Read the model definition and answer for the solid it produces. Units are mm, in the model's axes. A direction names the side the tool comes from. Round coordinates to 2 decimals unless told otherwise and drop trailing zeros. Order: outer loops, then holes, each group sorted by start corner. A loop starts at its lowest first (then second) coordinate and runs counter-clockwise, first axis right, second up. Notation, with made-up numbers: (-19, 12) - (35, 12) arc R25 ccw to (35, 37) - close; hole circle Ø8 at (8.5, 33). An arc over 180 degrees is marked (long way). Put each result on its own line as item: value. Start each with the question number.
Q1. Each of these flat-tipped pins is pushed along its axis until it touches: pin 1 Ø2.5 at (x, z) = (98, 2.5) entering from +Y (3 decimals); pin 2 Ø12 at (x, z) = (28.575, 44.45) entering from -Y; pin 3 Ø6.5 at (x, z) = (89.5, 5) entering from -Y (3 decimals); pin 4 Ø8 at (y, z) = (82, 16) entering from +X. Where does it stop, or does it pass through?
Q2. Section C-C on x = 81 is taken. Give the vertices of the cut face in (y, z) (1 decimal).
Q3. Which of the six approach directions +Z, -Z, +X, -X, +Y, -Y give full straight-line access (tool end or side, diameter ignored) to faces 1 (the face through (28.175, 79.514, 9.465)), 2 (the face through (88, 66.675, 4)), 3 (the face through (87, 22.225, 4))?
Q4. Section A-A on z = 29.5 is taken. Give the vertices of the cut face in (x, y), then the cut area to 3 significant figures.
Q5. For a pull along X with two mould halves and no side action, classify faces 4 (the face through (57.15, 6, 17)), 5 (the face through (29, 88.9, 29)), 6 (the face through (64.83, 38.17, 3.91)), 7 (the face through (27.95, 4.02, 73.02)) as pulls with the +X half, pulls with the -X half, needs draft (parallel to the pull), parting line crosses it, or undercut.
Q6. Find the intervals of material crossed by line 1 along X through (y, z) = (44, 3); line 2 along X through (y, z) = (3, 44); line 3 along Y through (x, z) = (18, 52.5), in increasing order. Write a range as from..to.
Q7. Section D-D on y = 44.45 is taken. Give the vertices of the cut face in (x, z), then the cut area to 3 significant figures.
from build123d import *

# Parameters (mm, degrees)
F0_W     = 57.15
F0_H     = 7.9375
F0_R     = 10.3251
F1_DEPTH = 7.9375
F2_DEPTH = 44.45
F3_DEPTH = 44.45
F4_W     = 28.575
F4_H     = 7.9375
F6_W     = 28.575
F6_H     = 7.9375
F8_R     = 9.92251
F9_DEPTH = 88.901
F10_R    = 5.08


with BuildPart() as f1:
    # F0 (on Top) → F1 (new body)
    with BuildSketch(Plane.XY):
        with Locations((28.575, 3.96875)):
            Rectangle(F0_W, F0_H)
        with BuildLine():
            Line((0, 80.9625), (0, 7.9375))
            Line((0, 7.9375), (57.15, 7.9375))
            Line((57.15, 7.9375), (57.15, 15.875))
            ThreePointArc((57.15, 15.875), (59.009872, 20.365128), (63.5, 22.225))
            Line((63.5, 22.225), (111.125, 22.225))
            ThreePointArc((111.125, 22.225), (133.35, 44.45), (111.125, 66.675))
            Line((111.125, 66.675), (63.5, 66.675))
            ThreePointArc((63.5, 66.675), (59.009872, 68.534872), (57.15, 73.025))
            Line((57.15, 73.025), (57.15, 80.9625))
            Line((57.15, 80.9625), (0, 80.9625))
        make_face()
        with Locations((73.025, 44.45)):
            Circle(F0_R, mode=Mode.SUBTRACT)
        with Locations((111.125, 44.45)):
            Circle(F0_R, mode=Mode.SUBTRACT)
        with Locations((28.575, 84.93125)):
            Rectangle(F0_W, F0_H)
    extrude(amount=F1_DEPTH)

    # F0 (on Top) → F2 (join)
    with BuildSketch(Plane.XY):
        with Locations((28.575, 3.96875)):
            Rectangle(F0_W, F0_H)
    extrude(amount=F2_DEPTH)

    # F0 (on Top) → F3 (join)
    with BuildSketch(Plane.XY):
        with Locations((28.575, 84.93125)):
            Rectangle(F0_W, F0_H)
    extrude(amount=F3_DEPTH)

    # F4 (on face) → F5 (revolve)
    with BuildSketch(Plane.XY.offset(44.45)):
        with Locations((14.2875, 3.96875)):
            Rectangle(F4_W, F4_H)
    revolve(axis=Axis((28.575, 3.96875, 44.45), (0, 1, 0)))

    # F6 (on face) → F7 (revolve)
    with BuildSketch(Plane.XY.offset(44.45)):
        with Locations((14.2875, 84.93125)):
            Rectangle(F6_W, F6_H)
    revolve(axis=Axis((28.575, 84.93125, 44.45), (0, 1, 0)))

    # F8 (on face) → F9 (cut, through all)
    with BuildSketch(Plane.XZ):
        with Locations((28.575, 44.45)):
            Circle(F8_R)
    extrude(amount=-F9_DEPTH, mode=Mode.SUBTRACT)

    # F10
    f10_edges = [f1.edges().sort_by_distance(p)[0] for p in [
        (28.575, 80.9625, 7.9375),
        (28.575, 7.9375, 7.9375),
    ]]
    fillet(f10_edges, radius=F10_R)


solid = f1.part
Findings:
1. pin 1: y = 66.675
1. pin 2: through
1. pin 3: y = 22.225
1. pin 4: x = 57.15
2. outline: (22.2, 0) - (37.9, 0) - (37.9, 7.9) - (22.2, 7.9) - close; (51, 0) - (66.7, 0) - (66.7, 7.9) - (51, 7.9) - close
3. face 1: +Z, +X, -X
3. face 2: +Z, -Z, +X, +Y
3. face 3: +Z, -Z, +X, -Y
4. outline: (0, 0) - (57.15, 0) - (57.15, 7.94) - (0, 7.94) - close; (0, 80.96) - (57.15, 80.96) - (57.15, 88.9) - (0, 88.9) - close
4. area: 907 mm2
5. face 4: pulls with the +X half
5. face 5: needs draft
5. face 6: undercut
5. face 7: parting line crosses it
6. line 1: 0..62.71, 83.34..100.81, 121.44..133.35
6. line 2: 0..18.66, 38.49..57.15
6. line 3: 0..7.94, 80.96..88.9
7. outline: (0, 0) - (62.7, 0) - (62.7, 7.94) - (0, 7.94) - close; (83.35, 0) - (100.8, 0) - (100.8, 7.94) - (83.35, 7.94) - close; (121.45, 0) - (133.35, 0) - (133.35, 7.94) - (121.45, 7.94) - close
7. area: 731 mm2
